Could you check a few things on this drawing? It's one solid part, dimensions in mm from its lowest x, y, z. A direction names the side the tool comes from. Give positions to 0.01 mm unless a question says otherwise; leave off trailing zeros. Order: outer loops, then holes, each group sorted by start corner. A loop starts at its lowest first (then second) coordinate and runs counter-clockwise, first axis right, second up.
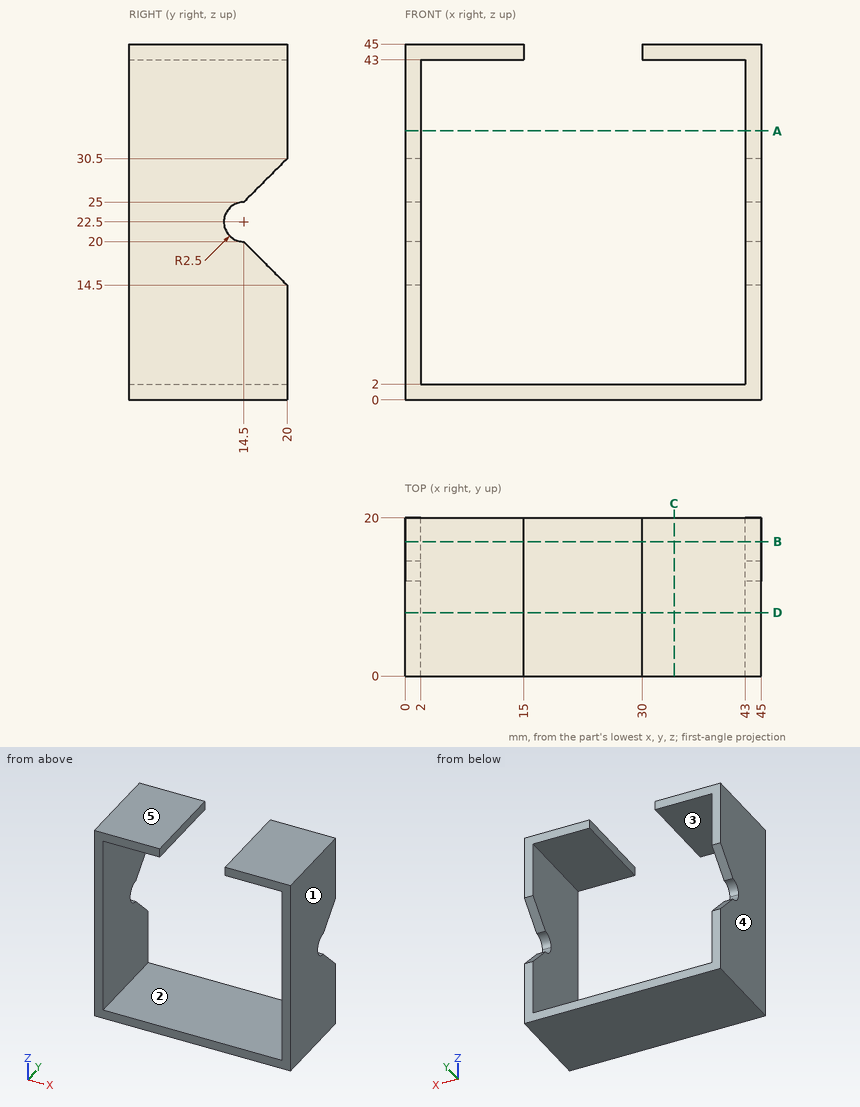
Item 1: Imagine slicing it at C-C on x = 34. List the corners of the cut face in (y, z) for me, then the cut area to 3 significant figures.
Findings:
outline: (0, 0) - (20, 0) - (20, 2) - (0, 2) - close; (0, 43) - (20, 43) - (20, 45) - (0, 45) - close
area: 80.0 mm2
Item 2: Imagine slicing it at B-B on y = 17. List the corners of the cut face in (x, z) for me.
Findings:
outline: (0, 0) - (45, 0) - (45, 17.5) - (43, 17.5) - (43, 2) - (2, 2) - (2, 17.5) - (0, 17.5) - close; (0, 27.5) - (2, 27.5) - (2, 43) - (15, 43) - (15, 45) - (0, 45) - close; (30, 43) - (43, 43) - (43, 27.5) - (45, 27.5) - (45, 45) - (30, 45) - close
Item 3: For the marked faces 1 and 2, which set-ups out of +Z, -Z, +X, -X, +Y, -Y let a thin tool reach every point of the face, with its end or its side?
Findings:
face 1: +Z, -Z, +X, +Y, -Y
face 2: +Y, -Y
Item 4: For pin 1 (8 mm diameter, centred on x = 33, z = 37.5, fed in from +Y), with a flat end and sliding along its axis, tell me the tip position at first contact or that it passes through.
Findings:
pin 1: passes through
Item 5: Imagine slicing it at A-A on z = 34. List the corners of the cut face in (x, y) for me.
Findings:
outline: (0, 0) - (2, 0) - (2, 20) - (0, 20) - close; (43, 0) - (45, 0) - (45, 20) - (43, 20) - close
Item 6: Imagine slicing it at D-D on y = 8. List the corners of the cut face in (x, z) for me.
Findings:
outline: (0, 0) - (45, 0) - (45, 45) - (30, 45) - (30, 43) - (43, 43) - (43, 2) - (2, 2) - (2, 43) - (15, 43) - (15, 45) - (0, 45) - close
Item 7: We'd pull the mould along Z, two halves only. Please class the marked faces 3, 4 and 5: +Z half, -Z half, draft (parallel to the pull), parting line (faces both ways), or undercut.
Findings:
face 3: undercut
face 4: draft
face 5: +Z half
Item 8: Please list where these lines run through material, in increasing order: line 1 along X through (y, z) = (3, 30.5); line 2 along Z through (x, y) = (25.5, 8).
Findings:
line 1: x = 0 to 2, 43 to 45
line 2: z = 0 to 2
